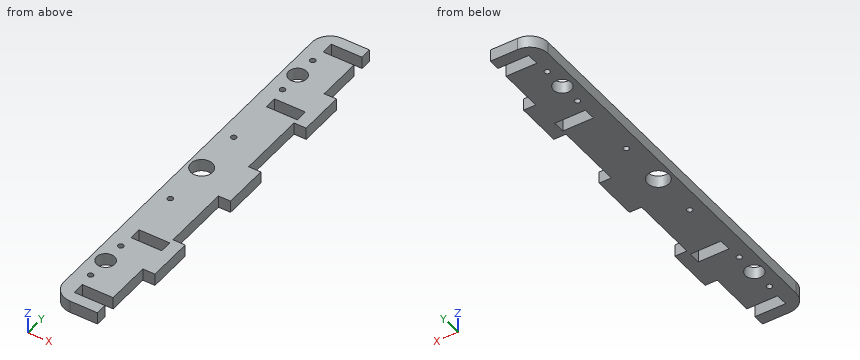
```python
from build123d import *

# Parameters (mm, degrees)
MODEL_R             = 4.75
MODEL_R_2           = 3.95
MODEL_R_3           = 1.2
MODEL_W             = 13.50000035
MODEL_H             = 5.350001156
MODEL_H_2           = 5.350008607
BOSS_EXTRUDE1_DEPTH = 5.35


with BuildPart() as part:
    # Model → Boss-Extrude1 (new body)
    with BuildSketch(Plane.XY):
        with BuildLine():
            Line((19.999999553, 174.99999702), (19.999999553, 180.000007153))
            Line((19.999999553, 180.000007153), (7.999999449, 180.000007153))
            ThreePointArc((7.999999449, 180.000007153), (2.343145556, 177.656861207), (0, 172.000007153))
            Line((0, 172.000007153), (0, 8.00000038))
            ThreePointArc((0, 8.00000038), (2.343145616, 2.343145885), (8, 0))
            Line((8, 0), (19.999999553, 0))
            Line((19.999999553, 0), (19.999999553, 4.999999888))
            Line((19.999999553, 4.999999888), (6.499999203, 4.999999888))
            Line((6.499999203, 4.999999888), (6.499999203, 10.350000113))
            Line((6.499999203, 10.350000113), (19.999999553, 10.350000113))
            Line((19.999999553, 10.350000113), (19.999999553, 29.99999933))
            Line((19.999999553, 29.99999933), (25.349999778, 29.99999933))
            Line((25.349999778, 29.99999933), (25.349999778, 50.000000745))
            Line((25.349999778, 50.000000745), (19.999999553, 50.000000745))
            Line((19.999999553, 50.000000745), (19.999999553, 79.999998212))
            Line((19.999999553, 79.999998212), (25.349999778, 79.999998212))
            Line((25.349999778, 79.999998212), (25.349999778, 100.00000149))
            Line((25.349999778, 100.00000149), (19.999999553, 100.00000149))
            Line((19.999999553, 100.00000149), (19.999999553, 129.999995232))
            Line((19.999999553, 129.999995232), (25.349999778, 129.999995232))
            Line((25.349999778, 129.999995232), (25.349999778, 150.000005961))
            Line((25.349999778, 150.000005961), (19.999999553, 150.000005961))
            Line((19.999999553, 150.000005961), (19.999999553, 169.650003314))
            Line((19.999999553, 169.650003314), (6.499999203, 169.650003314))
            Line((6.499999203, 169.650003314), (6.499999203, 174.99999702))
            Line((6.499999203, 174.99999702), (19.999999553, 174.99999702))
        make_face()
        with Locations((5.999999553, 90)):
            Circle(MODEL_R, mode=Mode.SUBTRACT)
        with Locations((5.999999553, 26.5)):
            Circle(MODEL_R_2, mode=Mode.SUBTRACT)
        with Locations((5.999999553, 153.5)):
            Circle(MODEL_R_2, mode=Mode.SUBTRACT)
        with Locations((6.159999553, 111)):
            Circle(MODEL_R_3, mode=Mode.SUBTRACT)
        with Locations((6.159999553, 69)):
            Circle(MODEL_R_3, mode=Mode.SUBTRACT)
        with Locations((5.999999553, 36.5)):
            Circle(MODEL_R_3, mode=Mode.SUBTRACT)
        with Locations((5.999999553, 16.5)):
            Circle(MODEL_R_3, mode=Mode.SUBTRACT)
        with Locations((5.999999553, 143.5)):
            Circle(MODEL_R_3, mode=Mode.SUBTRACT)
        with Locations((5.999999553, 163.5)):
            Circle(MODEL_R_3, mode=Mode.SUBTRACT)
        with Locations((13.249999378, 45.175001025)):
            Rectangle(MODEL_W, MODEL_H, mode=Mode.SUBTRACT)
        with Locations((13.249999378, 134.824998677)):
            Rectangle(MODEL_W, MODEL_H_2, mode=Mode.SUBTRACT)
    extrude(amount=BOSS_EXTRUDE1_DEPTH)


solid = part.part
```
The listing builds one solid part. Answer for the finished solid, in the listing's coordinates (mm). Give positions to 0.01 mm unless a question says otherwise; leave off trailing zeros. Order: outer loops, then holes, each group sorted by start corner. A loop starts at its lowest first (then second) coordinate and runs counter-clockwise, first axis right, second up.
Item 1: The part is cut by section C-C, the plane z = 3.1. Count the separate pieces of the cut face and the enclosed holes in it, and give its area (3 significant figures).
From the geometry:
separate pieces: 1
enclosed holes: 11
area: 3,410 mm2
Item 2: Given pin 1 Ø8.5 at (x, y) = (6, 90) entering from -Z; pin 2 Ø8 at (x, y) = (22.5, 85) entering from -Z; pin 3 Ø1.5 at (y, z) = (118, 1) entering from +X; pin 4 Ø1.6 at (y, z) = (171.5, 2) entering from +X, each flat-ended and moving along its own axis, determine where each tip first touches the part or whether it passes through.
From the geometry:
pin 1: passes through
pin 2: stops at z = 0
pin 3: stops at x = 20
pin 4: stops at x = 6.5
Item 3: The part is cut by section B-B, the plane y = 153.5. Give the vertices of the cut face in (x, z).
From the geometry:
outline: (0, 0) - (2.05, 0) - (2.05, 5.35) - (0, 5.35) - close; (9.95, 0) - (20, 0) - (20, 5.35) - (9.95, 5.35) - close
Item 4: The part is cut by section A-A, the plane x = 22. Give the vertices of the cut face in (y, z).
From the geometry:
outline: (30, 0) - (50, 0) - (50, 5.35) - (30, 5.35) - close; (80, 0) - (100, 0) - (100, 5.35) - (80, 5.35) - close; (130, 0) - (150, 0) - (150, 5.35) - (130, 5.35) - close
Item 5: Find the intervals of material crossed by probe 1 along Y at (x, z) = (21.75, 0.4); probe 2 along Y at (x, z) = (11.5, 5.1); probe 3 along Y at (x, z) = (4, 3.8), in increasing order.
From the geometry:
probe 1: y = 30 to 50, 80 to 100, 130 to 150
probe 2: y = 0 to 5, 10.35 to 42.5, 47.85 to 132.15, 137.5 to 169.65, 175 to 180
probe 3: y = 1.07 to 23.09, 29.91 to 85.69, 94.31 to 150.09, 156.91 to 178.93
Item 6: The part is cut by section D-D, the plane y = 128. Give the vertices of the cut face in (x, z), and give its area (3 significant figures).
From the geometry:
outline: (0, 0) - (20, 0) - (20, 5.35) - (0, 5.35) - close
area: 107 mm2
